Part model, mm, in its own coordinate system. A direction names the side the tool comes from. Give positions to 0.01 mm unless a question says otherwise; leave off trailing zeros. Order: outer loops, then holes, each group sorted by start corner. A loop starts at its lowest first (then second) coordinate and runs counter-clockwise, first axis right, second up.
from build123d import *

# Parameters (mm, degrees)
SKETCH_1_W          = 69
SKETCH_1_H          = 59
EXTRUDE_1_DEPTH     = 4
SKETCH_2_R          = 1.65
CUT_EXTRUDE_1_DEPTH = 4
SKETCH_3_R          = 3.25
CUT_EXTRUDE_2_DEPTH = 0.5
SKETCH_4_W          = 16
SKETCH_4_H          = 2.9
SKETCH_4_H_2        = 6.9
EXTRUDE_2_DEPTH     = 17
SKETCH_5_R          = 2.8
CUT_EXTRUDE_3_DEPTH = 57.249199994
FILLET_1_R          = 10
FILLET_2_R          = 4
CUT_EXTRUDE_4_DEPTH = 3.9
FILLET_3_R          = 1.5
SKETCH_7_R          = 5.3
CUT_EXTRUDE_5_DEPTH = 4
SKETCH_8_R          = 2.5
CUT_EXTRUDE_6_DEPTH = 10


# Some blends are built 0.0001 mm under size
with BuildPart() as part:
    # Эскиз1 → Бобышка-Вытянуть1 (new body)
    with BuildSketch(Plane(origin=(0, 0, 0), x_dir=(1, 0, 0), z_dir=(0, 1, 0))):
        Rectangle(SKETCH_1_W, SKETCH_1_H)
    extrude(amount=EXTRUDE_1_DEPTH)

    # Эскиз2 → Вырез-Вытянуть1 (cut)
    with BuildSketch(Plane(origin=(0, 4, 0), x_dir=(1, 0, 0), z_dir=(0, 1, 0))):
        with Locations(Location((-30.734773913, -25.856238371, 0), (0, 0, 270))):
            Circle(SKETCH_2_R)
        with Locations(Location((-30.734773913, 25.856238371, 0), (0, 0, 270))):
            Circle(SKETCH_2_R)
        with Locations(Location((0, 26, 0), (0, 0, 270))):
            Circle(SKETCH_2_R)
        with Locations(Location((30.734773913, 25.856238371, 0), (0, 0, 270))):
            Circle(SKETCH_2_R)
        with Locations(Location((30.734773913, -25.856238371, 0), (0, 0, 270))):
            Circle(SKETCH_2_R)
        with Locations(Location((0, -26, 0), (0, 0, 270))):
            Circle(SKETCH_2_R)
    extrude(amount=-CUT_EXTRUDE_1_DEPTH, mode=Mode.SUBTRACT)

    # Эскиз3 → Вырез-Вытянуть2 (cut)
    with BuildSketch(Plane(origin=(0, 4, 0), x_dir=(1, 0, 0), z_dir=(0, 1, 0))):
        with Locations(Location((-30.734773913, 25.856238371, 0), (0, 0, 270))):
            Circle(SKETCH_3_R)
        with Locations(Location((0, 26, 0), (0, 0, 270))):
            Circle(SKETCH_3_R)
        with Locations(Location((30.734773913, 25.856238371, 0), (0, 0, 270))):
            Circle(SKETCH_3_R)
        with Locations(Location((30.734773913, -25.856238371, 0), (0, 0, 270))):
            Circle(SKETCH_3_R)
        with Locations(Location((0, -26, 0), (0, 0, 270))):
            Circle(SKETCH_3_R)
        with Locations(Location((-30.734773913, -25.856238371, 0), (0, 0, 270))):
            Circle(SKETCH_3_R)
    extrude(amount=-CUT_EXTRUDE_2_DEPTH, mode=Mode.SUBTRACT)

    # Эскиз4 → Бобышка-Вытянуть2 (add)
    with BuildSketch(Plane(origin=(0, 4, 0), x_dir=(1, 0, 0), z_dir=(0, 1, 0))):
        with Locations((25, 8.2)):
            Rectangle(SKETCH_4_W, SKETCH_4_H)
        with Locations((25, 2)):
            Rectangle(SKETCH_4_W, SKETCH_4_H)
        with Locations((25, -6.2)):
            Rectangle(SKETCH_4_W, SKETCH_4_H_2)
    extrude(amount=EXTRUDE_2_DEPTH)

    # Эскиз5 → Вырез-Вытянуть3 (cut, through all)
    with BuildSketch(Plane(origin=(0, 0, -9.65), x_dir=(-1, 0, 0), z_dir=(0, 0, -1))):
        with Locations((-25, 15)):
            Circle(SKETCH_5_R)
    extrude(amount=-CUT_EXTRUDE_3_DEPTH, mode=Mode.SUBTRACT)

    # Скругление1
    # the kernel refuses this fillet: 10 mm, written as the material it takes off along each edge
    with BuildSketch(Plane(origin=(33, 21, -34.65), x_dir=(0, -1, 0), z_dir=(0, 0, 1)), Plane(origin=(17, 21, 18.25), x_dir=(0, -1, 0), z_dir=(0, 0, -1)), Plane(origin=(17, 21, 24.45), x_dir=(0, -1, 0), z_dir=(0, 0, -1)), Plane(origin=(33, 21, -28.45), x_dir=(0, -1, 0), z_dir=(0, 0, 1))) as fillet_1_piece_1:
        with BuildLine():
            CenterArc((FILLET_1_R, -FILLET_1_R), FILLET_1_R, 90, 90)
            Line((0, -FILLET_1_R), (0, 0))
            Line((0, 0), (FILLET_1_R, 0))
        make_face()
    extrude(amount=52.9, mode=Mode.SUBTRACT)
    with BuildSketch(Plane(origin=(33, 21, -22.25), x_dir=(0, -1, 0), z_dir=(0, 0, 1)), Plane(origin=(17, 21, 34.65), x_dir=(0, -1, 0), z_dir=(0, 0, -1))) as fillet_1_piece_2:
        with BuildLine():
            CenterArc((FILLET_1_R, -FILLET_1_R), FILLET_1_R, 90, 90)
            Line((0, -FILLET_1_R), (0, 0))
            Line((0, 0), (FILLET_1_R, 0))
        make_face()
    extrude(amount=56.9, mode=Mode.SUBTRACT)

    # Скругление2
    fillet_2_edges = [part.edges().sort_by_distance(p)[0] for p in [
        (25, 4, 9.65),
        (25, 4, -9.65),
    ]]
    fillet(fillet_2_edges, radius=FILLET_2_R)

    # Эскиз6 → Вырез-Вытянуть4 (cut)
    with BuildSketch(Plane.XY.offset(9.65)):
        Polygon((20.220834242, 14.649417644), (22.914030347, 10.685829867), (27.693196105, 11.036412222), (29.779165758, 15.350582356), (27.085969653, 19.314170133), (22.306803895, 18.963587778), align=None)
    extrude(amount=-CUT_EXTRUDE_4_DEPTH, mode=Mode.SUBTRACT)

    # Скругление3
    fillet_3_edges = [part.edges().sort_by_distance(p)[0] for p in [
        (33, 4, 8.2),
        (25, 4, 2.75),
        (17, 4, 8.2),
        (33, 4, -10.2),
        (17, 4, -10.2),
        (25, 4, -6.75),
        (33, 4, -2),
        (25, 4, -3.45),
        (17, 4, -2),
        (25, 4, -0.55),
    ]]
    fillet(fillet_3_edges, radius=FILLET_3_R - 0.0001)  # a hair under: the kernel refuses the full size

    # Эскиз7 → Вырез-Вытянуть5 (cut)
    with BuildSketch(Plane(origin=(0, 4, 0), x_dir=(1, 0, 0), z_dir=(0, 1, 0))):
        with Locations(Location((2.5, 6, 0), (0, 0, 270))):
            Circle(SKETCH_7_R)
    extrude(amount=-CUT_EXTRUDE_5_DEPTH, mode=Mode.SUBTRACT)

    # Эскиз8 → Вырез-Вытянуть6 (cut)
    with BuildSketch(Plane(origin=(0, 4, 0), x_dir=(1, 0, 0), z_dir=(0, 1, 0))):
        with Locations(Location((-26.5, 17.7, 0), (0, 0, 270))):
            Circle(SKETCH_8_R)
        with Locations(Location((-26.5, 5.9, 0), (0, 0, 270))):
            Circle(SKETCH_8_R)
        with Locations(Location((-26.5, -5.9, 0), (0, 0, 270))):
            Circle(SKETCH_8_R)
        with Locations(Location((-26.5, -17.7, 0), (0, 0, 270))):
            Circle(SKETCH_8_R)
        with Locations(Location((-16.5, 17.7, 0), (0, 0, 270))):
            Circle(SKETCH_8_R)
        with Locations(Location((-16.5, 5.9, 0), (0, 0, 270))):
            Circle(SKETCH_8_R)
        with Locations(Location((-16.5, -5.9, 0), (0, 0, 270))):
            Circle(SKETCH_8_R)
        with Locations(Location((-16.5, -17.7, 0), (0, 0, 270))):
            Circle(SKETCH_8_R)
    extrude(amount=-CUT_EXTRUDE_6_DEPTH, mode=Mode.SUBTRACT)


solid = part.part
Item 1: Band-saw the part on D-D on z = 26. List the corners of the cut face in (x, y), plus the area to 3 significant figures.
Item 2: Drop flat-ended pins along their axis: P1, Ø10.5, axis at x = 30.73, z = 25.86, coming from the +Y side; P2, Ø5, axis at y = 12.5, z = -1, coming from the +X side; P3, Ø12, axis at y = 15, z = -6, coming from the -X side. Give the stop position or say it passes through.
Item 3: Which spindle directions (+Z, -Z, +X, -X, +Y, -Y) get a long thin tool onto all of the face, cutting with end or side? Do faces 4 (the face through (25, 11, -3.45)), 5 (the face through (0.07, 1.77, -27.65)), 6 (the face through (25.27, 10.86, 7.73)), 7 (the face through (-1.4, 3.5, -24.6)), 8 (the face through (17, 8, -2)). Say none if no direction does.
Item 4: Band-saw the part on B-B on z = -17.7. List the corners of the cut face in (x, y), plus the area to 3 significant figures.
Item 5: Band-saw the part on C-C on y = 6.5. List the corners of the cut face in (x, z), plus the area to 3 significant figures.
Item 6: Band-saw the part on A-A on x = -16.5. List the corners of the cut face in (y, z).
Item 7: Drill centre lines: probe 1 along Z at (x, y) = (31.5, 10); probe 2 along X at (y, z) = (3.8, 26). Where is each one in solid material? Low to high.
Item 8: Pull direction Z, two halves, no side cores. Call faces 1 (the face through (33.45, 4.43, 7.54)), 2 (the face through (-18.94, 2.03, 17.16)), 3 (the face through (25, 11, -9.65)): released by +Z, released by -Z, zero draft, split by the parting line, or undercut.
Working result:
1. outline: (-34.5, 0) - (-32.38, 0) - (-32.38, 3.5) - (-33.98, 3.5) - (-33.98, 4) - (-34.5, 4) - close; (-29.09, 0) - (-1.65, 0) - (-1.65, 3.5) - (-3.25, 3.5) - (-3.25, 4) - (-27.49, 4) - (-27.49, 3.5) - (-29.09, 3.5) - close; (1.65, 0) - (29.09, 0) - (29.09, 3.5) - (27.49, 3.5) - (27.49, 4) - (3.25, 4) - (3.25, 3.5) - (1.65, 3.5) - close; (32.38, 0) - (34.5, 0) - (34.5, 4) - (33.98, 4) - (33.98, 3.5) - (32.38, 3.5) - close
1. area: 232 mm2
2. P1: stops at y = 4
2. P2: stops at x = 33
2. P3: stops at x = 17
3. face 4: +X, -X, +Y
3. face 5: +Y, -Y
3. face 6: +Z
3. face 7: +Y
3. face 8: +Z, -Z, -X, +Y
4. outline: (-34.5, 0) - (-29, 0) - (-29, 4) - (-34.5, 4) - close; (-24, 0) - (-19, 0) - (-19, 4) - (-24, 4) - close; (-14, 0) - (34.5, 0) - (34.5, 4) - (-14, 4) - close
4. area: 236 mm2
5. outline: (17, -9.94) - (33, -9.94) - (33, -6.75) - (17, -6.75) - close; (17, -3.45) - (33, -3.45) - (33, -0.55) - (17, -0.55) - close; (17, 2.75) - (33, 2.75) - (33, 9.94) - (17, 9.94) - close
5. area: 213 mm2
6. outline: (0, -29.5) - (4, -29.5) - (4, -20.2) - (0, -20.2) - close; (0, -15.2) - (4, -15.2) - (4, -8.4) - (0, -8.4) - close; (0, -3.4) - (4, -3.4) - (4, 3.4) - (0, 3.4) - close; (0, 8.4) - (4, 8.4) - (4, 15.2) - (0, 15.2) - close; (0, 20.2) - (4, 20.2) - (4, 29.5) - (0, 29.5) - close
7. probe 1: z = -9.65 to -6.75, -3.45 to -0.55, 2.75 to 9.65
7. probe 2: x = -34.5 to -33.98, -27.49 to -3.25, 3.25 to 27.49, 33.98 to 34.5
8. face 1: zero draft
8. face 2: undercut
8. face 3: released by -Z
